Study the drawing (mm; zero at the part's minimum x, y, z) and answer. A direction names the side the tool comes from. Coordinates: 2 decimals unless noted, no trailing zeros. Loops run counter-clockwise (first coordinate to the right, second up) from the corner with the lowest first, then second, coordinate; pieces in that order, holes last. Notation, with made-up numbers: (83, -11.75) - (111, -11.75) arc R7 ccw to (111, 1.25) - close; hole circle Ø10 at (-11, 50.5). An arc over 180 degrees is marked (long way). Use one line per item in the form item = value.
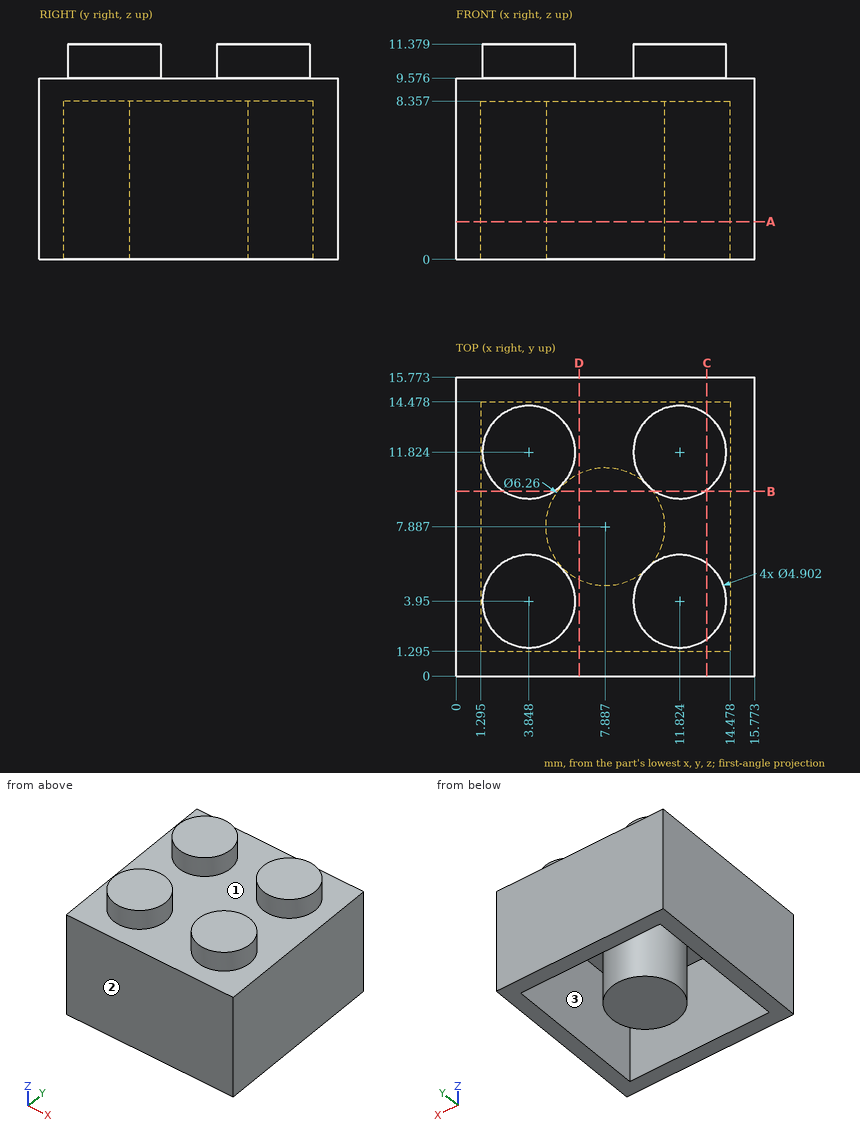
Item 1: The part is cut by section C-C on x = 13.25. Give the vertices of the cut face in (y, z) (1 decimal).
Results below:
outline = (0, 0) - (1.3, 0) - (1.3, 8.4) - (14.5, 8.4) - (14.5, 0) - (15.8, 0) - (15.8, 9.6) - (13.8, 9.6) - (13.8, 11.4) - (9.8, 11.4) - (9.8, 9.6) - (5.9, 9.6) - (5.9, 11.4) - (2, 11.4) - (2, 9.6) - (0, 9.6) - close
Item 2: Find the intervals of material crossed by L1, parallel to X at y = 4, z = 10.5 (1 decimal); L2, parallel to X at y = 9, z = 6.25 (1 decimal); L3, parallel to X at y = 9.5, z = 4.75 (1 decimal), in increasing order.
Results below:
L1 = 1.4 to 6.3, 9.4 to 14.3
L2 = 0 to 1.3, 5 to 10.8, 14.5 to 15.8
L3 = 0 to 1.3, 5.2 to 10.6, 14.5 to 15.8
Item 3: The part is cut by section B-B on y = 9.75. Give the vertices of the cut face in (x, z) (1 decimal).
Results below:
outline = (0, 0) - (1.3, 0) - (1.3, 8.4) - (5.4, 8.4) - (5.4, 0) - (10.4, 0) - (10.4, 8.4) - (14.5, 8.4) - (14.5, 0) - (15.8, 0) - (15.8, 9.6) - (13.1, 9.6) - (13.1, 11.4) - (10.5, 11.4) - (10.5, 9.6) - (5.2, 9.6) - (5.2, 11.4) - (2.5, 11.4) - (2.5, 9.6) - (0, 9.6) - close
Item 4: Which of the six approach directions +Z, -Z, +X, -X, +Y, -Y give full straight-line access (tool end or side, diameter ignored) to the marked faces 1, 2 and 3?
Results below:
face_1 = +Z
face_2 = +Z, -Z, +X, -X, -Y
face_3 = -Z
Item 5: The part is cut by section D-D on x = 6.5. Give the vertices of the cut face in (y, z) (1 decimal).
Results below:
outline = (0, 0) - (1.3, 0) - (1.3, 8.4) - (5.1, 8.4) - (5.1, 0) - (10.7, 0) - (10.7, 8.4) - (14.5, 8.4) - (14.5, 0) - (15.8, 0) - (15.8, 9.6) - (0, 9.6) - close
Item 6: Each of these flat-tipped pins is pushed along its axis until it touches: P1, Ø1, axis at x = 7.5, y = 13.5, coming from the -Z side; P2, Ø8, axis at x = 3, y = 7, coming from the -Z side. Where does it stop, or does it pass through?
Results below:
P1 = 8.36
P2 = 0
Item 7: The part is cut by section A-A on z = 2. Give the vertices of the cut face in (x, y) (1 decimal).
Results below:
outline = (0, 0) - (15.8, 0) - (15.8, 15.8) - (0, 15.8) - close; circle Ø6.3 at (7.9, 7.9); hole (1.3, 1.3) - (14.5, 1.3) - (14.5, 14.5) - (1.3, 14.5) - close
